Can you work these out from the model? Positions are in its coordinate system, mm. Face numbers are marked on the shaded views. A direction names the side the tool comes from. Round coordinates to 2 decimals unless told otherwise and drop trailing zeros. Loops run counter-clockwise (first coordinate to the right, second up) from the corner with the lowest first, then second, coordinate; pieces in that order, holes last.
from build123d import *

# Parameters (mm, degrees)
SKETCH_2_W      = 124
SKETCH_2_H      = 124
EXTRUDE_1_DEPTH = 2
SKETCH_6_W      = 124
SKETCH_6_H      = 124
SKETCH_6_W_2    = 120
SKETCH_6_H_2    = 120
EXTRUDE_3_DEPTH = 42
SKETCH_7_R      = 2
EXTRUDE_4_DEPTH = 2


with BuildPart() as part:
    # 草图2 → 凸台-拉伸1 (new body)
    with BuildSketch(Plane(origin=(0, 0, 0), x_dir=(1, 0, 0), z_dir=(0, 1, 0))):
        with Locations((62, 62)):
            Rectangle(SKETCH_2_W, SKETCH_2_H)
    extrude(amount=EXTRUDE_1_DEPTH)

    # 草图6 → 凸台-拉伸3 (add)
    with BuildSketch(Plane(origin=(0, 2, 0), x_dir=(1, 0, 0), z_dir=(0, 1, 0))):
        with Locations((62, 62)):
            Rectangle(SKETCH_6_W, SKETCH_6_H)
        with Locations((62, 62)):
            Rectangle(SKETCH_6_W_2, SKETCH_6_H_2, mode=Mode.SUBTRACT)
    extrude(amount=EXTRUDE_3_DEPTH)

    # 草图7 → 凸台-拉伸4 (add)
    with BuildSketch(Plane(origin=(0, 2, 0), x_dir=(1, 0, 0), z_dir=(0, 1, 0))):
        with Locations(Location((6.5, 6.5, 0), (0, 0, 90))):
            Circle(SKETCH_7_R)
        with Locations(Location((117.5, 6.5, 0), (0, 0, 90))):
            Circle(SKETCH_7_R)
        with Locations(Location((6.5, 117.5, 0), (0, 0, 90))):
            Circle(SKETCH_7_R)
        with Locations(Location((117.5, 117.5, 0), (0, 0, 90))):
            Circle(SKETCH_7_R)
    extrude(amount=EXTRUDE_4_DEPTH)


solid = part.part
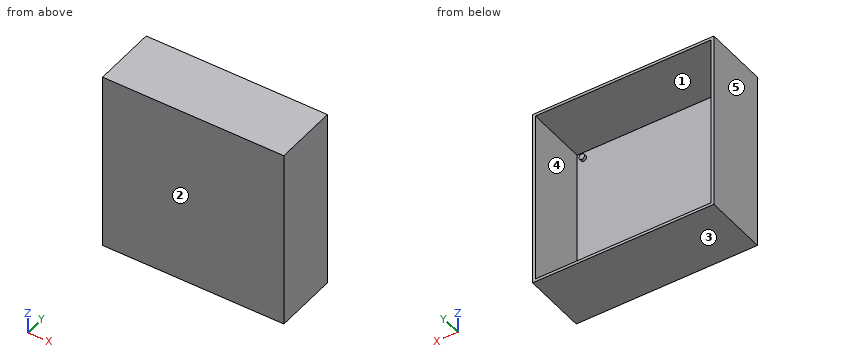
(1) If we section it at B-B, the plane z = -109: List the corners of the cut face in (x, y) for me, then the cut area to 3 significant figures.
Worked answers:
outline: (0, 0) - (124, 0) - (124, 44) - (122, 44) - (122, 2) - (2, 2) - (2, 44) - (0, 44) - close
area: 416 mm2
(2) If we mould it in two halves opening along Z, with no side actions, what happens to the marked faces 3, 4 and 5? For each: released by +Z, released by -Z, zero draft, split by the parting line, or undercut.
Worked answers:
face 3: released by -Z
face 4: undercut
face 5: zero draft
(3) For the marked faces 1 and 2, which set-ups out of +Z, -Z, +X, -X, +Y, -Y let a thin tool reach every point of the face, with its end or its side?
Worked answers:
face 1: +Y
face 2: +Z, -Z, +X, -X, -Y
(4) If I drill on line 1 (Z direction, x = 119.5, y = 28.5); line 2 (X direction, y = 21.5, z = -75.5); line 3 (Y direction, x = 116.5, z = -12.5), over which ranges is the centre line in solid material (lowest first)?
Worked answers:
line 1: z = -124 to -122, -2 to 0
line 2: x = 0 to 2, 122 to 124
line 3: y = 0 to 2
(5) If we section it at C-C, the plane x = 6.5: List the corners of the cut face in (y, z) for me, then the cut area to 3 significant figures.
Worked answers:
outline: (0, -124) - (44, -124) - (44, -122) - (2, -122) - (2, -119.5) - (4, -119.5) - (4, -115.5) - (2, -115.5) - (2, -8.5) - (4, -8.5) - (4, -4.5) - (2, -4.5) - (2, -2) - (44, -2) - (44, 0) - (0, 0) - close
area: 432 mm2
(6) Will these pins go through, and if not, where does the flat tip stop? P1, Ø1.2, axis at x = 118, z = -117, coming from the +Y side; P2, Ø4, axis at y = 12.5, z = -106.5, coming from the -X side; P3, Ø8, axis at x = 14, z = -44.5, coming from the +Y side.
Worked answers:
P1: stops at y = 4
P2: stops at x = 0
P3: stops at y = 2
(7) If we section it at A-A, the plane y = 22: List the corners of the cut face in (x, z) for me, then the cut area to 3 significant figures.
Worked answers:
outline: (0, -124) - (124, -124) - (124, 0) - (0, 0) - close; hole (2, -122) - (122, -122) - (122, -2) - (2, -2) - close
area: 976 mm2
